from build123d import *

# Parameters (mm, degrees)
TUBE001_R       = 10
TUBE001_R_2     = 1.7
TUBE001_DEPTH   = 2.5
CHAMFER002_SIZE = 2
FILLET001_R     = 2.4


with BuildPart() as part:
    # Tube001 → Tube001 (new body)
    with BuildSketch(Plane.XY):
        Circle(TUBE001_R)
        Circle(TUBE001_R_2, mode=Mode.SUBTRACT)
    extrude(amount=TUBE001_DEPTH)

    # Chamfer002
    chamfer002_edges = [part.edges().sort_by_distance(p)[0] for p in [
        (-1.7, 0, 0),
    ]]
    chamfer(chamfer002_edges, length=CHAMFER002_SIZE)

    # Fillet001
    fillet001_edges = [part.edges().sort_by_distance(p)[0] for p in [
        (-10, 0, 0),
    ]]
    fillet(fillet001_edges, radius=FILLET001_R)


with BuildPart() as part_1:
    # Fillet001 placement: moved
    add(part.part.moved(Location((0, 0, 50))))


solid = part_1.part
Work out the finished part from the listing and answer in its coordinate system (mm). Give positions to 0.01 mm unless a question says otherwise; leave off trailing zeros. Loops run counter-clockwise (first coordinate to the right, second up) from the corner with the lowest first, then second, coordinate; pieces in that order, holes last. Notation, with made-up numbers: (-35, 68) -> (-14, 68) arc R13 cw to (-14, 93) -> close; hole circle Ø5 at (10.25, 41.25). An arc over 180 degrees is marked (long way). Use a Markdown table: item, result. Add a question column.
1. Section A-A on y = 0 is taken. Determine the outline of the cut face in (x, z).
2. Find the intervals of material crossed by probe 1 along Y at (x, z) = (0, 52.35); probe 2 along Y at (x, z) = (-0.5, 51.7); probe 3 along X at (y, z) = (1.5, 51.85), in increasing order.
3. Flat-ended cylindrical pins translate along their axes: pin 1 Ø1.5 at (x, z) = (-5, 50.5) entering from -Y; pin 2 Ø1 at (y, z) = (-2.5, 52) entering from +X; pin 3 Ø6 at (x, y) = (8, 6) entering from -Z; pin 4 Ø4 at (x, y) = (0, 0) entering from -Z. Find the tip coordinate at first contact, or state that the pin passes through.
4. Section C-C on z = 50.4 is taken. Determine the outline of the cut face in (x, y).
5. Determine the mould class of faces 1 (the flat face through (2, 0, 52.5)), 2 (the conical face through (-0.396, -1.782, 51.875)) for opening direction X: released by +X, released by -X, zero draft, split by the parting line, or undercut.
Results below:
| question | item | result |
|---|---|---|
| 1 | outline | (-10, 52.4) arc R2.4 ccw to (-7.6, 50) -> (-3.7, 50) -> (-1.7, 52) -> (-1.7, 52.5) -> (-10, 52.5) -> close; (1.7, 52) -> (3.7, 50) -> (7.6, 50) arc R2.4 ccw to (10, 52.4) -> (10, 52.5) -> (1.7, 52.5) -> close |
| 2 | probe 1 | y = -10 to -1.7, 1.7 to 10 |
| 2 | probe 2 | y = -9.88 to -1.94, 1.94 to 9.88 |
| 2 | probe 3 | x = -9.82 to -1.08, 1.08 to 9.82 |
| 3 | pin 1 | stops at y = -8.47 |
| 3 | pin 2 | stops at x = 9.78 |
| 3 | pin 3 | stops at z = 50 |
| 3 | pin 4 | stops at z = 51.7 |
| 4 | outline | circle Ø17.85 at (0, 0); hole circle Ø6.6 at (0, 0) |
| 5 | face 1 | zero draft |
| 5 | face 2 | undercut |
